```python
from build123d import *

# Parameters (mm, degrees)
F0_R          = 44.45
F0_R_2        = 16.51
F1_DEPTH      = 38.1
F1_DEPTH_BACK = 38.1
F6_R          = 3.175
F6_R_2        = 1.9685
F7_DEPTH      = 48.26
F8_R          = 6.35
F9_DEPTH      = 7.62
F10_R         = 3.429
F11_DEPTH     = 68.58
F12_R         = 6.35
F13_DEPTH     = 76.2


with BuildPart() as f1:
    # F0 (on Top) → F1 (new body, two sides)
    with BuildSketch(Plane.XY) as f1_sk:
        with Locations((-96.7949852347, 47.625)):
            Circle(F0_R)
        with Locations((-96.7949852347, 47.625)):
            Circle(F0_R_2, mode=Mode.SUBTRACT)
        with Locations((-96.7949852347, 47.625)):
            Circle(F0_R_2)
        with BuildLine():
            ThreePointArc((-88.1051627648, 52.1100670498), (-87.4115771175, 50.37826953), (-87.0594782396, 48.5462733292))
            ThreePointArc((-87.0594782396, 48.5462733292), (-85.6757800173, 47.965243489), (-85.103715896, 46.5778145407))
            ThreePointArc((-85.103715896, 46.5778145407), (-85.8323827306, 45.0488259953), (-87.478931514, 44.6517889292))
            ThreePointArc((-87.478931514, 44.6517889292), (-88.2130581693, 42.9367840447), (-89.2595036018, 41.3923956038))
            ThreePointArc((-89.2595036018, 41.3923956038), (-88.839336444, 40.7569162622), (-88.6919210429, 40.0094919292))
            ThreePointArc((-88.6919210429, 40.0094919292), (-90.1000831422, 38.1224270954), (-92.309918185, 38.9351775301))
            ThreePointArc((-92.309918185, 38.9351775301), (-94.0417157047, 38.2415918827), (-95.8737119056, 37.8894930048))
            ThreePointArc((-95.8737119056, 37.8894930048), (-98.0529677671, 35.9450498204), (-99.7681963056, 38.3089462792))
            ThreePointArc((-99.7681963056, 38.3089462792), (-101.48320119, 39.0430729345), (-103.0275896309, 40.089518367))
            ThreePointArc((-103.0275896309, 40.089518367), (-105.9434851899, 40.2555560033), (-105.4848077047, 43.1399329502))
            ThreePointArc((-105.4848077047, 43.1399329502), (-106.178393352, 44.87173047), (-106.5304922299, 46.7037266708))
            ThreePointArc((-106.5304922299, 46.7037266708), (-108.4749354144, 48.8829825323), (-106.1110389555, 50.5982110708))
            ThreePointArc((-106.1110389555, 50.5982110708), (-105.3769123002, 52.3132159553), (-104.3304668677, 53.8576043962))
            ThreePointArc((-104.3304668677, 53.8576043962), (-104.1644292314, 56.7734999551), (-101.2800522845, 56.3148224699))
            ThreePointArc((-101.2800522845, 56.3148224699), (-99.5482547647, 57.0084081173), (-97.7162585639, 57.3605069952))
            ThreePointArc((-97.7162585639, 57.3605069952), (-95.7414309138, 59.3162590358), (-93.7792997754, 57.3477693387))
            ThreePointArc((-93.7792997754, 57.3477693387), (-93.7899471678, 57.1433056087), (-93.8217741639, 56.9410537208))
            ThreePointArc((-93.8217741639, 56.9410537208), (-92.1067692795, 56.2069270655), (-90.5623808386, 55.160481633))
            ThreePointArc((-90.5623808386, 55.160481633), (-88.4202847093, 55.5757742752), (-87.210977164, 53.7595641919))
            ThreePointArc((-87.210977164, 53.7595641919), (-87.4489020941, 52.8214265806), (-88.1051627648, 52.1100670498))
        make_face(mode=Mode.SUBTRACT)
        with BuildLine():
            ThreePointArc((-87.478931514, 44.6517889292), (-89.0293967369, 46.7886116136), (-87.0594782396, 48.5462733292))
            ThreePointArc((-87.0594782396, 48.5462733292), (-87.4115771175, 50.37826953), (-88.1051627648, 52.1100670498))
            ThreePointArc((-88.1051627648, 52.1100670498), (-90.7124690483, 52.524684387), (-90.5623808386, 55.160481633))
            ThreePointArc((-90.5623808386, 55.160481633), (-92.1067692795, 56.2069270655), (-93.8217741639, 56.9410537208))
            ThreePointArc((-93.8217741639, 56.9410537208), (-95.9585968484, 55.3905884978), (-97.7162585639, 57.3605069952))
            ThreePointArc((-97.7162585639, 57.3605069952), (-99.5482547647, 57.0084081173), (-101.2800522845, 56.3148224699))
            ThreePointArc((-101.2800522845, 56.3148224699), (-101.0424845928, 55.8008459714), (-100.9610494266, 55.2405080708))
            ThreePointArc((-100.9610494266, 55.2405080708), (-102.1821250936, 53.4194234719), (-104.3304668677, 53.8576043962))
            ThreePointArc((-104.3304668677, 53.8576043962), (-105.3769123002, 52.3132159553), (-106.1110389555, 50.5982110708))
            ThreePointArc((-106.1110389555, 50.5982110708), (-104.988766028, 49.9120186247), (-104.5492545734, 48.6721854593))
            ThreePointArc((-104.5492545734, 48.6721854593), (-105.1303256251, 47.2757495806), (-106.5304922299, 46.7037266708))
            ThreePointArc((-106.5304922299, 46.7037266708), (-106.178393352, 44.87173047), (-105.4848077047, 43.1399329502))
            ThreePointArc((-105.4848077047, 43.1399329502), (-103.4723556943, 43.221010878), (-102.4419933055, 41.4904358081))
            ThreePointArc((-102.4419933055, 41.4904358081), (-102.5942832222, 40.7312433534), (-103.0275896309, 40.089518367))
            ThreePointArc((-103.0275896309, 40.089518367), (-101.48320119, 39.0430729345), (-99.7681963056, 38.3089462792))
            ThreePointArc((-99.7681963056, 38.3089462792), (-97.6377069641, 39.8600832689), (-95.8736706941, 37.9022306613))
            ThreePointArc((-95.8736706941, 37.9022306613), (-95.873680997, 37.8958617997), (-95.8737119056, 37.8894930048))
            ThreePointArc((-95.8737119056, 37.8894930048), (-94.0417157047, 38.2415918827), (-92.309918185, 38.9351775301))
            ThreePointArc((-92.309918185, 38.9351775301), (-91.8953008477, 41.5424838136), (-89.2595036018, 41.3923956038))
            ThreePointArc((-89.2595036018, 41.3923956038), (-88.2130581693, 42.9367840447), (-87.478931514, 44.6517889292))
        make_face()
    extrude(amount=F1_DEPTH)
    extrude(f1_sk.sketch, amount=-F1_DEPTH_BACK)

    # F2 (on Top) → F3 (revolve, cut)
    with BuildSketch(Plane.XY):
        with BuildLine():
            Line((-107.66797587, -48.3024583081), (-131.1163690465, -6.7040645718))
            Line((-131.1163690465, -6.7040645718), (-154.564762223, 34.8943291645))
            ThreePointArc((-154.564762223, 34.8943291645), (-172.7147627828, -30.1524577483), (-107.66797587, -48.3024583081))
        make_face()
        with BuildLine():
            Line((-174.4341057324, 105.0050152593), (-126.6846434119, 104.5127225599))
            Line((-126.6846434119, 104.5127225599), (-78.9351810914, 104.0204298605))
            ThreePointArc((-78.9351810914, 104.0204298605), (-126.1923507125, 152.2621848804), (-174.4341057324, 105.0050152593))
        make_face()
        with BuildLine():
            Line((-8.2828741018, 86.1724430488), (-32.5839432458, 45.0663420119))
            Line((-32.5839432458, 45.0663420119), (-56.8850123899, 3.960240975))
            ThreePointArc((-56.8850123899, 3.960240975), (8.5221577911, 20.7652728678), (-8.2828741018, 86.1724430488))
        make_face()
    revolve(axis=Axis((-150.5593745721, 104.7588689096, 0), (0.9999468571, -0.0103093629, 0)), mode=Mode.SUBTRACT)

    # F2 (on Top) → F4 (revolve, cut)
    with BuildSketch(Plane.XY):
        with BuildLine():
            Line((-8.2828741018, 86.1724430488), (-32.5839432458, 45.0663420119))
            Line((-32.5839432458, 45.0663420119), (-56.8850123899, 3.960240975))
            ThreePointArc((-56.8850123899, 3.960240975), (8.5221577911, 20.7652728678), (-8.2828741018, 86.1724430488))
        make_face()
    revolve(axis=Axis((-44.7344778179, 24.5132914934, 0), (-0.5089015988, -0.8608246992, 0)), mode=Mode.SUBTRACT)

    # F2 (on Top) → F5 (revolve, cut)
    with BuildSketch(Plane.XY):
        with BuildLine():
            Line((-107.66797587, -48.3024583081), (-131.1163690465, -6.7040645718))
            Line((-131.1163690465, -6.7040645718), (-154.564762223, 34.8943291645))
            ThreePointArc((-154.564762223, 34.8943291645), (-172.7147627828, -30.1524577483), (-107.66797587, -48.3024583081))
        make_face()
    revolve(axis=Axis((-119.3921724583, -27.5032614399, 0), (-0.4910452583, 0.8711340622, 0)), mode=Mode.SUBTRACT)

    # F6 (on face) → F7 (cut)
    with BuildSketch(Plane.XY.offset(38.1)):
        with Locations((-102.9295494266, 55.2405080708)):
            Circle(F6_R)
        with Locations((-102.9295494266, 55.2405080708)):
            Circle(F6_R_2, mode=Mode.SUBTRACT)
        with Locations((-95.7477997754, 57.3477693387)):
            Circle(F6_R)
        with Locations((-95.7477997754, 57.3477693387)):
            Circle(F6_R_2, mode=Mode.SUBTRACT)
        with Locations((-89.179477164, 53.7595641919)):
            Circle(F6_R)
        with Locations((-89.179477164, 53.7595641919)):
            Circle(F6_R_2, mode=Mode.SUBTRACT)
        with Locations((-87.072215896, 46.5778145407)):
            Circle(F6_R)
        with Locations((-87.072215896, 46.5778145407)):
            Circle(F6_R_2, mode=Mode.SUBTRACT)
        with Locations((-90.6604210429, 40.0094919292)):
            Circle(F6_R)
        with Locations((-90.6604210429, 40.0094919292)):
            Circle(F6_R_2, mode=Mode.SUBTRACT)
        with Locations((-97.8421706941, 37.9022306613)):
            Circle(F6_R)
        with BuildLine():
            ThreePointArc((-95.8736706941, 37.9022306613), (-95.873680997, 37.8958617997), (-95.8737119056, 37.8894930048))
            ThreePointArc((-95.8737119056, 37.8894930048), (-99.8106603912, 37.9085995228), (-95.8736706941, 37.9022306613))
        make_face(mode=Mode.SUBTRACT)
        with Locations((-104.4104933055, 41.4904358081)):
            Circle(F6_R)
        with Locations((-104.4104933055, 41.4904358081)):
            Circle(F6_R_2, mode=Mode.SUBTRACT)
        with Locations((-106.5177545734, 48.6721854593)):
            Circle(F6_R)
        with Locations((-106.5177545734, 48.6721854593)):
            Circle(F6_R_2, mode=Mode.SUBTRACT)
    extrude(amount=-F7_DEPTH, mode=Mode.SUBTRACT)

    # F8 (on face) → F9 (cut)
    with BuildSketch(Plane.XY.offset(38.1)):
        with Locations((-96.7949852347, 47.625)):
            Circle(F8_R)
    extrude(amount=-F9_DEPTH, mode=Mode.SUBTRACT)

    # F10 (on face) → F11 (cut, through all)
    with BuildSketch(Plane.XY.offset(30.48)):
        with Locations((-96.7949852347, 47.625)):
            Circle(F10_R)
    extrude(amount=-F11_DEPTH, mode=Mode.SUBTRACT)

    # F12 (on face) → F13 (cut, through all)
    with BuildSketch(Plane.XY.offset(38.1)):
        with Locations((-127.8890646346, 48.8640254414)):
            Circle(F12_R)
        with BuildLine():
            ThreePointArc((-76.7834769385, 79.3022345884), (-85.5434026681, 77.325191035), (-83.5663591148, 68.5652653054))
            Line((-83.5663591148, 68.5652653054), (-76.7834769385, 79.3022345884))
        make_face()
        with BuildLine():
            Line((-76.7834769385, 79.3022345884), (-83.5663591148, 68.5652653054))
            ThreePointArc((-83.5663591148, 68.5652653054), (-77.1100486093, 68.3723584434), (-73.8249180267, 73.9337499469))
            ThreePointArc((-73.8249180267, 73.9337499469), (-74.6135265232, 76.9986193642), (-76.7834769385, 79.3022345884))
        make_face()
        with Locations((-82.3209730429, 20.0772246117)):
            Circle(F12_R)
    extrude(amount=-F13_DEPTH, mode=Mode.SUBTRACT)


solid = f1.part
```
The listing builds one solid part. Answer for the finished solid, in the listing's coordinates (mm). A direction names the side the tool comes from. Coordinates: 2 decimals unless noted, no trailing zeros. Write each loop counter-clockwise with the first axis right and the second up, starting at its lowest first coordinate (ties: lowest second). Pieces come first, ordered by that corner, then holes. Notation, with made-up numbers: (28.25, -15.75) -> (83.25, -15.75) arc R23 ccw to (83.25, 23.25) -> close; hole circle Ø10 at (88.25, 33.5). An arc over 180 degrees is marked (long way). Write each question's results on one line, items separated by ' | '. Start each with the question number.
1) For a pull along Y with two mould halves and no side action, classify faces 1 (the cylindrical face through (-132.93, 45, 0.53)), 2 (the flat face through (-89, 48, -38.1)), 3 (the cylindrical face through (-72.712, 84.985, 0.533)) as +Y half, -Y half, draft (parallel to the pull), parting line (faces both ways), or undercut.
2) A cutting plane is placed at D-D (x = -125.5). Determine the outline of the cut face in (y, z), then the cut area to 3 significant figures.
3) A cutting plane is placed at A-A (x = -62). Determine the outline of the cut face in (y, z), then the cut area to 3 significant figures.
4) A tool of negligible diameter and unlimited length cuts with its end or side. For faces 4 (the flat face through (-103, 53, -10.16)), 5 (the cylindrical face through (-93.63, 46.31, -3.33)), from which of +Z, -Z, +X, -X, +Y, -Y can it reach the whole face along a straight path? Write none if from no direction.
5) Straight lines are drawn through the part: probe 1 along Y at (x, z) = (-80, 14); probe 2 along Y at (x, z) = (-82.5, 24); probe 3 along Z at (x, y) = (-67.5, 42). For each, find the intervals that lie inside material, in ascending order.
6) Flat-ended cylindrical pins translate along their axes: pin 1 Ø10 at (x, y) = (-127.89, 48.86) entering from -Z; pin 2 Ø3 at (x, z) = (-83, -0.5) entering from -Y; pin 3 Ø6 at (x, z) = (-78.5, -4) entering from +Y; pin 4 Ø6.5 at (x, y) = (-96, 49.5) entering from +Z. Find the tip coordinate at first contact, or state that the pin passes through.
7) A cutting plane is placed at B-B (z = 17). Count the separate pieces of the cut face and the enclosed holes in it, then the cut area to 3 significant figures.
Values follow:
1) face 1: undercut | face 2: draft | face 3: +Y half
2) outline: (21.53, -38.1) -> (42.98, -38.1) -> (42.98, 38.1) -> (21.53, 38.1) arc R47.42 cw to start; (54.75, -38.1) -> (75.75, -38.1) arc R47.74 cw to (75.75, 38.1) -> (54.75, 38.1) -> close | area: 1,200 mm²
3) outline: (19.96, -38.1) -> (75.29, -38.1) -> (75.29, -22.4) arc R37.62 cw to (19.96, -28.01) -> close; (19.96, 28.01) arc R37.62 cw to (75.29, 22.4) -> (75.29, 38.1) -> (19.96, 38.1) -> close | area: 482 mm²
4) face 4: +Z | face 5: +Z, -Z
5) probe 1: 6.47 to 14.17, 25.99 to 67.59, 80.28 to 88.78 | probe 2: 5.54 to 13.73, 26.42 to 68.02, 79.84 to 89.71 | probe 3: -38.1 to -32.43, 32.43 to 38.1
6) pin 1: through | pin 2: y = 4.91 | pin 3: y = 89.36 | pin 4: z = 30.48
7) separate pieces: 1 | enclosed holes: 12 | area: 2,380 mm²
